```python
from build123d import *

# Parameters (mm, degrees)
ESQUISSE1_W        = 56.6
ESQUISSE1_H        = 29.6
ESQUISSE1_W_2      = 55
ESQUISSE1_H_2      = 28
BOSS_EXTRU_1_DEPTH = 48
CONG_1_R           = 1


with BuildPart() as part:
    # Esquisse1 → Boss.-Extru.1 (new body)
    with BuildSketch(Plane.XY):
        Rectangle(ESQUISSE1_W, ESQUISSE1_H)
        Rectangle(ESQUISSE1_W_2, ESQUISSE1_H_2, mode=Mode.SUBTRACT)
    extrude(amount=BOSS_EXTRU_1_DEPTH)

    # Congé1
    cong_1_edges = [part.edges().sort_by_distance(p)[0] for p in [
        (27.5, -14, 24),
        (27.5, 14, 24),
        (-27.5, 14, 24),
        (-27.5, -14, 24),
        (-28.3, 14.8, 24),
        (28.3, 14.8, 24),
        (28.3, -14.8, 24),
        (-28.3, -14.8, 24),
    ]]
    fillet(cong_1_edges, radius=CONG_1_R)


solid = part.part
```
Work out the finished part from the listing and answer in its coordinate system (mm). A direction names the side the tool comes from. Give positions to 0.01 mm unless a question says otherwise; leave off trailing zeros. Order: outer loops, then holes, each group sorted by start corner. A loop starts at its lowest first (then second) coordinate and runs counter-clockwise, first axis right, second up. Notation, with made-up numbers: (69.25, 55) -> (94.25, 55) arc R22 cw to (94.25, 79) -> close; hole circle Ø8 at (86.5, 28). An arc over 180 degrees is marked (long way). Answer as CSV lines item,"result". Start each with the question number.
(1) Section C-C, the plane z = 45 is taken. Write down the section's boundary in (x, y), plus the area to 3 significant figures.
(2) Section B-B, the plane x = -7 is taken. Write down the section's boundary in (y, z).
(3) For a pull along X with two mould halves and no side action, classify faces 1 (the flat face through (0, 14, 24)), 2 (the flat face through (0, -14.8, 24)), 3 (the flat face through (-28.3, 0, 24)) as released by +X, released by -X, zero draft, split by the parting line, or undercut.
(4) Consider line 1 along X through (y, z) = (-1, 25); line 2 along Y through (x, z) = (-26, 17.5). Determine where each line is inside the solid, lowest interval first.
(5) Section A-A, the plane y = -2.5 is taken. Write down the section's boundary in (x, z).
(6) Which of the six approach directions +Z, -Z, +X, -X, +Y, -Y give full straight-line access (tool end or side, diameter ignored) to faces 4 (the flat face through (27.5, 0, 24)), 5 (the flat face through (28.3, 0, 24))?
Entries:
1,outline,"(-28.3, -13.8) arc R1 ccw to (-27.3, -14.8) -> (27.3, -14.8) arc R1 ccw to (28.3, -13.8) -> (28.3, 13.8) arc R1 ccw to (27.3, 14.8) -> (-27.3, 14.8) arc R1 ccw to (-28.3, 13.8) -> close; hole (-27.5, -13) arc R1 ccw to (-26.5, -14) -> (26.5, -14) arc R1 ccw to (27.5, -13) -> (27.5, 13) arc R1 ccw to (26.5, 14) -> (-26.5, 14) arc R1 ccw to (-27.5, 13) -> close"
1,area,"135 mm²"
2,outline,"(-14.8, 0) -> (-14, 0) -> (-14, 48) -> (-14.8, 48) -> close; (14, 0) -> (14.8, 0) -> (14.8, 48) -> (14, 48) -> close"
3,face 1,"undercut"
3,face 2,"zero draft"
3,face 3,"released by -X"
4,line 1,"-28.3 to -27.5, 27.5 to 28.3"
4,line 2,"-14.8 to -14, 14 to 14.8"
5,outline,"(-28.3, 0) -> (-27.5, 0) -> (-27.5, 48) -> (-28.3, 48) -> close; (27.5, 0) -> (28.3, 0) -> (28.3, 48) -> (27.5, 48) -> close"
6,face 4,"+Z, -Z"
6,face 5,"+Z, -Z, +X, +Y, -Y"
